Geometry check sheet. Reference: drawing and pictorial views, mm from the part's lowest x, y, z. A direction names the side the tool comes from. Coordinates: 2 decimals unless noted, no trailing zeros. Loops run counter-clockwise (first coordinate to the right, second up) from the corner with the lowest first, then second, coordinate; pieces in that order, holes last.
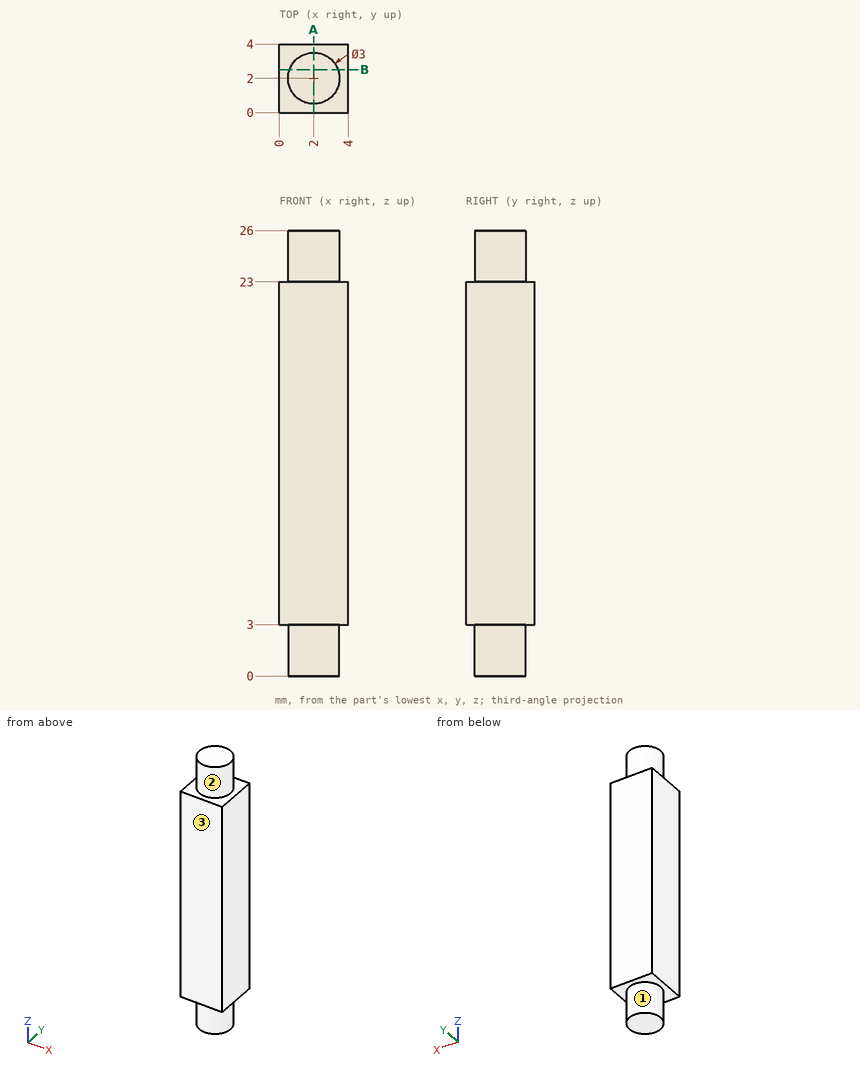
1) Material ranges on probe 1 along Z at (x, y) = (2.3, 3.6); probe 2 along X at (y, z) = (1.75, 24.75); probe 3 along X at (y, z) = (2.9, 24.25), recorded low to high.
Data:
probe 1: z = 3 to 23
probe 2: x = 0.52 to 3.48
probe 3: x = 0.8 to 3.2
2) Section check B-B on y = 2.5. Record the cut outline in (x, z).
Data:
outline: (0, 3) - (0.59, 3) - (0.59, 0) - (3.41, 0) - (3.41, 3) - (4, 3) - (4, 23) - (3.41, 23) - (3.41, 26) - (0.59, 26) - (0.59, 23) - (0, 23) - close
3) Access from +Z, -Z, +X, -X, +Y, -Y to the whole of each face (thin tool, end or side, straight path). Record for the marked faces 1, 2 and 3.
Data:
face 1: -Z
face 2: +Z
face 3: +Z, -Z, +X, -X, -Y
4) Section check A-A on x = 2. Record the cut outline in (y, z), and give its area (3 significant figures).
Data:
outline: (0, 3) - (0.5, 3) - (0.5, 0) - (3.5, 0) - (3.5, 3) - (4, 3) - (4, 23) - (3.5, 23) - (3.5, 26) - (0.5, 26) - (0.5, 23) - (0, 23) - close
area: 98.0 mm2
